from build123d import *

# Parameters (mm, degrees)
BOSS_EXTRUDE1_DEPTH = 0.8128
SKETCH2_W           = 19.05
SKETCH2_H           = 24.2062
BOSS_EXTRUDE2_DEPTH = 1.8796
BOSS_EXTRUDE3_DEPTH = 0.8636
SKETCH4_W           = 1.9812
SKETCH4_H           = 19.75
BOSS_EXTRUDE4_DEPTH = 1.778
SKETCH5_W           = 0.508
SKETCH5_H           = 0.508
BOSS_EXTRUDE5_DEPTH = 4.064
SKETCH6_R           = 0.762


with BuildPart() as part:
    # Sketch1 → Boss-Extrude1 (new body)
    with BuildSketch(Plane(origin=(0, 0, 0), x_dir=(1, 0, 0), z_dir=(0, 1, 0))):
        Polygon((0, 0), (24.384, 0), (24.384, 26.162), (16.7259, 32.9438), (7.6581, 32.9438), (0, 26.162), align=None)
    extrude(amount=BOSS_EXTRUDE1_DEPTH)

    # Sketch2 → Boss-Extrude2 (add)
    with BuildSketch(Plane(origin=(0, 0, 0), x_dir=(-1, 0, 0), z_dir=(0, -1, 0))):
        with Locations((-12.192, 12.8651)):
            Rectangle(SKETCH2_W, SKETCH2_H)
    extrude(amount=BOSS_EXTRUDE2_DEPTH)

    # Sketch3 → Boss-Extrude3 (add)
    with BuildSketch(Plane(origin=(0, 0.8128, 0), x_dir=(1, 0, 0), z_dir=(0, 1, 0))):
        Polygon((4.3307, 7.342503403), (10.517503403, 13.832203403), (17.007203403, 7.6454), (10.8204, 1.1557), align=None)
    extrude(amount=BOSS_EXTRUDE3_DEPTH)

    # Sketch4 → Boss-Extrude4 (add)
    with BuildSketch(Plane(origin=(0, 0, 0), x_dir=(-1, 0, 0), z_dir=(0, -1, 0))):
        with Locations((-1.016, 16.2616)):
            Rectangle(SKETCH4_W, SKETCH4_H)
        with Locations((-23.368, 16.2616)):
            Rectangle(SKETCH4_W, SKETCH4_H)
    extrude(amount=BOSS_EXTRUDE4_DEPTH)

    # Sketch5 → Boss-Extrude5 (add)
    with BuildSketch(Plane(origin=(0, -1.778, 0), x_dir=(-1, 0, 0), z_dir=(0, -1, 0))):
        with Locations((-23.368, 25.2913)):
            Rectangle(SKETCH5_W, SKETCH5_H)
        with Locations((-23.368, 23.2847)):
            Rectangle(SKETCH5_W, SKETCH5_H)
        with Locations((-23.368, 21.2781)):
            Rectangle(SKETCH5_W, SKETCH5_H)
        with Locations((-23.368, 19.2715)):
            Rectangle(SKETCH5_W, SKETCH5_H)
        with Locations((-23.368, 17.2649)):
            Rectangle(SKETCH5_W, SKETCH5_H)
        with Locations((-23.368, 15.2583)):
            Rectangle(SKETCH5_W, SKETCH5_H)
        with Locations((-23.368, 13.2517)):
            Rectangle(SKETCH5_W, SKETCH5_H)
        with Locations((-23.368, 11.2451)):
            Rectangle(SKETCH5_W, SKETCH5_H)
        with Locations((-23.368, 9.2385)):
            Rectangle(SKETCH5_W, SKETCH5_H)
        with Locations((-23.368, 7.2319)):
            Rectangle(SKETCH5_W, SKETCH5_H)
        with Locations((-1.016, 7.2319)):
            Rectangle(SKETCH5_W, SKETCH5_H)
        with Locations((-1.016, 9.2385)):
            Rectangle(SKETCH5_W, SKETCH5_H)
        with Locations((-1.016, 11.2451)):
            Rectangle(SKETCH5_W, SKETCH5_H)
        with Locations((-1.016, 13.2517)):
            Rectangle(SKETCH5_W, SKETCH5_H)
        with Locations((-1.016, 15.2583)):
            Rectangle(SKETCH5_W, SKETCH5_H)
        with Locations((-1.016, 17.2649)):
            Rectangle(SKETCH5_W, SKETCH5_H)
        with Locations((-1.016, 19.2715)):
            Rectangle(SKETCH5_W, SKETCH5_H)
        with Locations((-1.016, 21.2781)):
            Rectangle(SKETCH5_W, SKETCH5_H)
        with Locations((-1.016, 23.2847)):
            Rectangle(SKETCH5_W, SKETCH5_H)
        with Locations((-1.016, 25.2913)):
            Rectangle(SKETCH5_W, SKETCH5_H)
    extrude(amount=BOSS_EXTRUDE5_DEPTH)

    # Sweep2: sweep along a curve in space
    with BuildLine() as sweep2_path:
        add(Edge.make_bspline(
            [(15.1892, 0.8128, -29.337), (20.622976284, 5.000023383, -30.448552109), (16.989821563, 2.292008104, -17.951240105)],
            knots=[0, 0, 0, 1, 1, 1], degree=2))
    # Sketch6 → Sweep2 (sweep)
    with BuildSketch(Plane(origin=(0, 0.8128, 0), x_dir=(1, 0, 0), z_dir=(0, 1, 0))):
        with Locations((15.1892, 29.337)):
            Circle(SKETCH6_R)
    sweep(path=sweep2_path.line)


solid = part.part
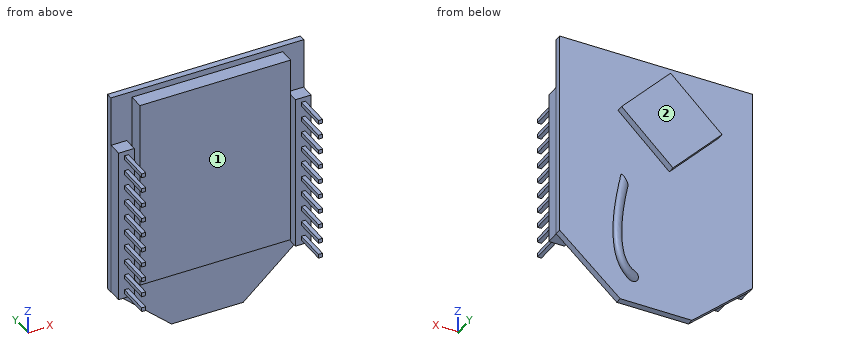
Can you work these out from the model? Positions are in its coordinate system, mm. Face numbers are marked on the shaded views. Coordinates: 2 decimals unless noted, no trailing zeros. Order: outer loops, then holes, each group sorted by start corner. A loop starts at its lowest first (then second) coordinate and runs counter-clockwise, first axis right, second up. Notation, with made-up numbers: M -8.5,84.25 L 42.5,84.25 A17 ccw 42.5,106.25 Z; hole C -1.75,50 d5. An arc over 180 degrees is marked long. Write item = value, one per line.
(1) I need wall thicknesses on line 1 along Y through (x, z) = (12.5, -18); line 2 along Y through (x, z) = (14.5, -28); line 3 along Z through (x, y) = (13, -1.25). Which ranges of each line are inside material? Lowest first, please. Write a range as [from, to].
Results are:
line_1 = [-1.88, 0.81]
line_2 = [0, 0.81]
line_3 = [-24.97, -0.76]
(2) Suppose I cut it at D-D on y = -3.75. State how many separate pieces and enclosed holes the cut face has, plus the area to 3 significant figures.
Results are:
separate_pieces = 20
enclosed_holes = 0
area = 5.16 mm2
(3) For pin 1 Ø5 at (x, z) = (10.5, -25) entering from -Y; pin 2 Ø3 at (y, z) = (-3, -7) entering from +X; pin 3 Ø4 at (x, z) = (17, -27) entering from -Y, each with a flat end and sliding along its axis, tell me the tip position at first contact or that it passes through.
Results are:
pin_1 = -1.88
pin_2 = 24.36
pin_3 = 0
(4) If we mould it in two halves opening along X, with no side actions, what happens to the marked faces 1 and 2? For each: pulls with the +X half, pulls with the -X half, needs draft (parallel to the pull), parting line crosses it, or undercut.
Results are:
face_1 = undercut
face_2 = needs draft
(5) Suppose I cut it at C-C on x = 19.5. Please give me the cut outline in (y, z).
Results are:
outline = M -1.88,-24.97 L 0,-24.97 L 0,-30.49 L 0.81,-30.49 L 0.81,0 L 0,0 L 0,-0.76 L -1.88,-0.76 Z
(6) Suppose I cut it at A-A on y = -0.5. Please give me the cut outline in (x, z), plus the area to 3 significant figures.
Results are:
outline = M 0.03,-26.14 L 2.01,-26.14 L 2.01,-6.39 L 0.03,-6.39 Z; M 2.67,-24.97 L 21.72,-24.97 L 21.72,-0.76 L 2.67,-0.76 Z; M 22.38,-26.14 L 24.36,-26.14 L 24.36,-6.39 L 22.38,-6.39 Z
area = 539 mm2
